Input: part model. Units: mm. Frame: model coordinates. Face numbers are marked on the shaded views. A direction names the side the tool comes from. Coordinates: 2 decimals unless noted, no trailing zeros. Write each loop counter-clockwise with the first axis right and the second up, starting at its lowest first coordinate (ties: lowest second). Pieces come first, ordered by that corner, then holes. Notation, with made-up numbers: (51, 30.25) - (109, 30.25) arc R4 ccw to (109, 36.25) - close; hole circle Ø5 at (43.25, 76). An arc over 180 degrees is marked (long way). Put each result on its own line as item: value. Start each with the question number.
1. Pull-direction query (X, two-part tool) for the marked faces 3, 4 and 5; classes: released by +X, released by -X, zero draft, split by the parting line, or undercut.
2. Access query for the marked faces 1 and 2. Directions: +Z, -Z, +X, -X, +Y, -Y. A direction counts if a zero-diameter tool reaches every point of the face in a straight line with its end or side. Return the directions, or none.
3. Cut plane D-D, the plane x = -7. Return loops of the section in (y, z), and give its area (3 significant figures).
4. Cut plane C-C, the plane x = -75. Return loops of the section in (y, z), and give its area (3 significant figures).
5. Line query: line 1 (X direction, y = -11.5, z = -3); line 2 (X direction, y = -18.3, z = 20); line 3 (X direction, y = -8.55, z = -10). Output: solid intervals per line, ascending.
6. Pin query (flat end, axial travel): pin 1 (16 mm diameter, centred on x = 38.5, z = -3, fed in from -Y); pin 2 (10 mm diameter, centred on x = 32, y = -2, fed in from +Z); pin 3 (2.5 mm diameter, centred on x = -75.5, z = 0, fed in from +Y); pin 4 (8 mm diameter, centred on x = 40, z = 0, fed in from +Y). Return the tip coordinate at first contact, or that it passes through.
7. Cut plane A-A, the plane x = 65. Return loops of the section in (y, z), and give its area (3 significant figures).
8. Cut plane B-B, the plane z = 10. Return loops of the section in (x, y).
from build123d import *

# Parameters (mm, degrees)
SKETCH1_W           = 300
SKETCH1_H           = 30
SKETCH1_W_2         = 10
SKETCH1_H_2         = 10
BOSS_EXTRUDE1_DEPTH = 20
SKETCH12_W          = 10
SKETCH12_H          = 10
CUT_EXTRUDE5_DEPTH  = 10
SKETCH14_W          = 10
SKETCH14_H          = 10
CUT_EXTRUDE6_DEPTH  = 10
SKETCH3_W           = 20
SKETCH3_H           = 30
CUT_EXTRUDE1_DEPTH  = 10
SKETCH5_R           = 2.5
CUT_EXTRUDE3_DEPTH  = 154.378616502
CUT_EXTRUDE4_REACH  = 154.398
SKETCH7_R           = 5
SKETCH15_W          = 30
SKETCH15_H          = 30
CUT_EXTRUDE7_DEPTH  = 5
SKETCH16_R          = 2.5
CUT_EXTRUDE8_DEPTH  = 5


with BuildPart() as part:
    # Sketch1 → Boss-Extrude1 (new body)
    with BuildSketch(Plane(origin=(0, 0, 0), x_dir=(1, 0, 0), z_dir=(0, 1, 0))):
        Rectangle(SKETCH1_W, SKETCH1_H)
        with Locations((-145, -20)):
            Rectangle(SKETCH1_W_2, SKETCH1_H_2)
        with Locations((-145, 20)):
            Rectangle(SKETCH1_W_2, SKETCH1_H_2)
        with Locations((145, 20)):
            Rectangle(SKETCH1_W_2, SKETCH1_H_2)
        with Locations((145, -20)):
            Rectangle(SKETCH1_W_2, SKETCH1_H_2)
    extrude(amount=-BOSS_EXTRUDE1_DEPTH)

    # Sketch12 → Cut-Extrude5 (cut)
    with BuildSketch(Plane.XY.offset(25)):
        with Locations((-145, -10)):
            Rectangle(SKETCH12_W, SKETCH12_H)
        with Locations((145, -10)):
            Rectangle(SKETCH12_W, SKETCH12_H)
    extrude(amount=-CUT_EXTRUDE5_DEPTH, mode=Mode.SUBTRACT)

    # Sketch14 → Cut-Extrude6 (cut)
    with BuildSketch(Plane(origin=(0, 0, -25), x_dir=(-1, 0, 0), z_dir=(0, 0, -1))):
        with Locations((-145, -10)):
            Rectangle(SKETCH14_W, SKETCH14_H)
        with Locations((145, -10)):
            Rectangle(SKETCH14_W, SKETCH14_H)
    extrude(amount=-CUT_EXTRUDE6_DEPTH, mode=Mode.SUBTRACT)

    # Sketch3 → Cut-Extrude1 (cut)
    with BuildSketch(Plane.XZ.offset(20)):
        with Locations((-40, 0)):
            Rectangle(SKETCH3_W, SKETCH3_H)
        with Locations((40, 0)):
            Rectangle(SKETCH3_W, SKETCH3_H)
    extrude(amount=-CUT_EXTRUDE1_DEPTH, mode=Mode.SUBTRACT)

    # Sketch5 → Cut-Extrude3 (cut, through all)
    with BuildSketch(Plane(origin=(0, 0, 0), x_dir=(1, 0, 0), z_dir=(0, 1, 0))):
        with Locations(Location((145, -20, 0), (0, 0, 270))):
            Circle(SKETCH5_R)
        with Locations(Location((145, 20, 0), (0, 0, 270))):
            Circle(SKETCH5_R)
        with Locations(Location((-145, 20, 0), (0, 0, 270))):
            Circle(SKETCH5_R)
        with Locations(Location((-145, -20, 0), (0, 0, 90))):
            Circle(SKETCH5_R)
    extrude(amount=-CUT_EXTRUDE3_DEPTH, mode=Mode.SUBTRACT)

    # Sketch7 → Cut-Extrude4 (cut, up to next)
    with BuildSketch(Plane.XZ.offset(10), mode=Mode.PRIVATE) as cut_extrude4_sk1:
        with Locations(Location((-40, 0, 0), (0, 0, 270))):
            Circle(SKETCH7_R)
    cut_extrude4_tool1 = extrude(cut_extrude4_sk1.sketch, amount=-CUT_EXTRUDE4_REACH, mode=Mode.PRIVATE) & part.part
    # Sketch7 → Cut-Extrude4 (cut, up to next)
    with BuildSketch(Plane.XZ.offset(10), mode=Mode.PRIVATE) as cut_extrude4_sk2:
        with Locations(Location((40, 0, 0), (0, 0, 90))):
            Circle(SKETCH7_R)
    cut_extrude4_tool2 = extrude(cut_extrude4_sk2.sketch, amount=-CUT_EXTRUDE4_REACH, mode=Mode.PRIVATE) & part.part
    add(cut_extrude4_tool1.solids().sort_by_distance((-40, -10, 0))[0], mode=Mode.SUBTRACT)
    add(cut_extrude4_tool2.solids().sort_by_distance((40, -10, 0))[0], mode=Mode.SUBTRACT)

    # Sketch15 → Cut-Extrude7 (cut)
    with BuildSketch(Plane(origin=(0, 0, 0), x_dir=(1, 0, 0), z_dir=(0, 1, 0))):
        with Locations((-65, 0)):
            Rectangle(SKETCH15_W, SKETCH15_H)
    cut_extrude7 = extrude(amount=-CUT_EXTRUDE7_DEPTH, mode=Mode.SUBTRACT)

    # Mirror1: Cut-Extrude7 across plane
    add(cut_extrude7.mirror(Plane(origin=(0, 0, 0), x_dir=(0, 0, 1), z_dir=(1, 0, 0))), mode=Mode.SUBTRACT)

    # Sketch16 → Cut-Extrude8 (cut)
    with BuildSketch(Plane(origin=(0, -5, 0), x_dir=(1, 0, 0), z_dir=(0, 1, 0))):
        with Locations(Location((-65, 10, 0), (0, 0, 270))):
            Circle(SKETCH16_R)
        with Locations(Location((-75, 0, 0), (0, 0, 270))):
            Circle(SKETCH16_R)
        with Locations(Location((-65, -10, 0), (0, 0, 270))):
            Circle(SKETCH16_R)
        with Locations(Location((-55, 0, 0), (0, 0, 270))):
            Circle(SKETCH16_R)
    cut_extrude8 = extrude(amount=-CUT_EXTRUDE8_DEPTH, mode=Mode.SUBTRACT)

    # Mirror2: Cut-Extrude8 across plane
    add(cut_extrude8.mirror(Plane(origin=(0, 0, 0), x_dir=(0, 0, 1), z_dir=(1, 0, 0))), mode=Mode.SUBTRACT)


solid = part.part
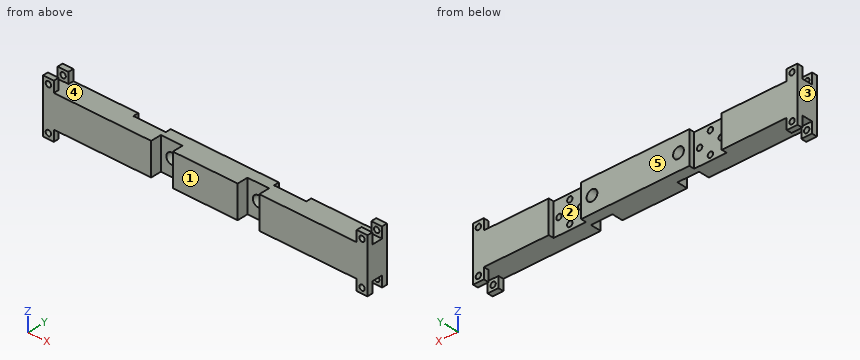
Report:
1. face 3: released by -X
1. face 4: undercut
1. face 5: zero draft
2. face 1: +Z, -Z, +X, -X, -Y
2. face 2: +Z, -Z, +Y
3. outline: (-20, -15) - (0, -15) - (0, 15) - (-20, 15) - close
3. area: 600 mm^2
4. outline: (-20, -15) - (-5, -15) - (-5, -2.5) - (-10, -2.5) - (-10, 2.5) - (-5, 2.5) - (-5, 15) - (-20, 15) - close
4. area: 425 mm^2
5. line 1: x = -150 to -50, -30 to 30, 50 to 150
5. line 2: x = -150 to -147.5, -142.5 to -140, 140 to 142.5, 147.5 to 150
5. line 3: x = -150 to -67.5, -62.5 to 62.5, 67.5 to 150
6. pin 1: stops at y = -10
6. pin 2: stops at z = 15
6. pin 3: stops at y = -10
6. pin 4: passes through
7. outline: (-20, -15) - (-5, -15) - (-5, -12.5) - (-10, -12.5) - (-10, -7.5) - (-5, -7.5) - (-5, 7.5) - (-10, 7.5) - (-10, 12.5) - (-5, 12.5) - (-5, 15) - (-20, 15) - close
7. area: 400 mm^2
8. outline: (-150, -20) - (-50, -20) - (-50, -10) - (-30, -10) - (-30, -20) - (30, -20) - (30, -10) - (50, -10) - (50, -20) - (150, -20) - (150, 0) - (80, 0) - (80, -5) - (67.5, -5) - (67.5, -10) - (62.5, -10) - (62.5, -5) - (50, -5) - (50, 0) - (-50, 0) - (-50, -5) - (-62.5, -5) - (-62.5, -10) - (-67.5, -10) - (-67.5, -5) - (-80, -5) - (-80, 0) - (-150, 0) - close
